Geometry check sheet. Reference: the model listing, model coordinates, mm. A direction names the side the tool comes from. Round coordinates to 2 decimals unless told otherwise and drop trailing zeros. Order: outer loops, then holes, each group sorted by start corner. A loop starts at its lowest first (then second) coordinate and runs counter-clockwise, first axis right, second up.
Autodesk Inventor part; units mm, degrees
ref_plane "YZ Plane" through (0, 0, 0) normal (1, 0, 0) x (0, 1, 0)
ref_plane "XZ Plane" through (0, 0, 0) normal (0, 1, 0) x (-1, 0, 0)
ref_plane "XY Plane" through (0, 0, 0) normal (0, 0, 1) x (1, 0, 0)
sketch "Sketch1" plane through (0, 0, 0) normal (0, 0, 1) x (1, 0, 0)
  line L0 (-107.95, -107.95) -> (107.95, -107.95)
  line L1 (107.95, -107.95) -> (107.95, 107.95)
  line L2 (107.95, 107.95) -> (-107.95, 107.95)
  line L3 (-107.95, 107.95) -> (-107.95, -107.95)
  line L4 (-107.95, -107.95) -> (107.95, 107.95) construction
  point P0 (0, 0)
  point P1 (0, 0)
  dimension "d0" = 215.9
  dimension "d1" = 215.9
extrude "Extrusion1" add sketch "Sketch1" along normal blind 6.35
sketch "Sketch3" plane through (0, 0, 6.35) normal (0, 0, 1) x (1, 0, 0)
  circle A0 centre (0, 0) radius 57.785
  dimension "d44" = 115.57
extrude "Extrusion3" cut sketch "Sketch3" against normal through all
sketch "Sketch5" plane through (0, 0, 6.35) normal (0, 0, 1) x (1, 0, 0)
  line L0 (-95.25, -95.25) -> (95.25, -95.25) construction
  line L1 (95.25, -95.25) -> (95.25, 95.25) construction
  line L2 (95.25, 95.25) -> (-95.25, 95.25) construction
  line L3 (-95.25, 95.25) -> (-95.25, -95.25) construction
  line L4 (-95.25, -95.25) -> (95.25, 95.25) construction
  point P0 (0, 0)
  point P1 (0, 0)
  point P2 (0, 0)
  dimension "d15" = 190.5
  dimension "d16" = 190.5
hole "Hole1" at (-95.25, 95.25, 6.35) at (95.25, 95.25, 6.35) at (95.25, -95.25, 6.35) at (-95.25, -95.25, 6.35) direction (0, 0, -1) diameter 4.4958 end through all counterbore diameter 7.9502 counterbore depth 4.1656
sketch "Sketch6" plane through (0, 0, 0) normal (0, 0, -1) x (-1, 0, 0)
  line L0 (-63.5, -63.5) -> (63.5, -63.5) construction
  line L1 (63.5, -63.5) -> (63.5, 63.5) construction
  line L2 (63.5, 63.5) -> (-63.5, 63.5) construction
  line L3 (-63.5, 63.5) -> (-63.5, -63.5) construction
  line L4 (-63.5, -63.5) -> (63.5, 63.5) construction
  point P0 (0, 0)
  point P1 (0, 0)
  dimension "d24" = 127
  dimension "d25" = 127
hole "Hole2" at (63.5, 63.5, 0) at (-63.5, 63.5, 0) at (-63.5, -63.5, 0) at (63.5, -63.5, 0) direction (0, 0, 1) diameter 3.302 end through all
sketch "Sketch7" plane through (0, 0, 6.35) normal (0, 0, 1) x (1, 0, 0)
  line L0 (-91.44, -91.44) -> (91.44, -91.44) construction
  line L1 (91.44, -91.44) -> (91.44, 91.44) construction
  line L2 (91.44, 91.44) -> (-91.44, 91.44) construction
  line L3 (-91.44, 91.44) -> (-91.44, -91.44) construction
  line L4 (-91.44, -91.44) -> (91.44, 91.44) construction
  line L5 (-151.13, 0) -> (151.13, 0) construction
  line L6 (0, -151.13) -> (0, 151.13) construction
  point P0 (0, 0)
  point P1 (0, 0)
  point P2 (-68.58, 91.44)
  point P3 (0, 91.44)
  point P4 (68.58, 91.44)
  point P5 (91.44, 68.58)
  point P6 (91.44, 0)
  point P7 (91.44, -68.58)
  point P8 (68.58, -91.44)
  point P9 (0, -91.44)
  point P10 (-68.58, -91.44)
  point P11 (-91.44, -68.58)
  point P12 (-91.44, 0)
  point P13 (-91.44, 68.58)
  dimension "d33" = 182.88
  dimension "d34" = 182.88
  dimension "d35" = 22.86
  dimension "d36" = 22.86
hole "Hole3" at (-68.58, 91.44, 6.35) at (0, 91.44, 6.35) at (68.58, 91.44, 6.35) at (91.44, 68.58, 6.35) at (91.44, 0, 6.35) at (91.44, -68.58, 6.35) at (68.58, -91.44, 6.35) at (0, -91.44, 6.35) at (-68.58, -91.44, 6.35) at (-91.44, -68.58, 6.35) at (-91.44, 0, 6.35) at (-91.44, 68.58, 6.35) direction (0, 0, -1) diameter 3.302 end through all
equation "\"d15\" = d16"
equation "\"d25\" = d24"
properties part number "J002448" material "ALUMINUM, 6061-T651"
(1) Draft check along Y on faces 3 (the flat face through (107.95, -2, 3)), 4 (the flat face through (-2, -107.95, 3)), 5 (the flat face through (-93.5, -97, 2.184)). Enter one of: released by +Y, released by -Y, zero draft, split by the parting line, or undercut.
Returned:
face 3: zero draft
face 4: released by -Y
face 5: undercut
(2) Set-up check for faces 1 (the cylindrical face through (-91.37, -94.39, 4.24)), 2 (the flat face through (-107.95, 2, 3)): record each of +Z, -Z, +X, -X, +Y, -Y from which the full face is reachable in a straight line by a thin tool's end or side.
Returned:
face 1: +Z
face 2: +Z, -Z, -X, +Y, -Y
(3) Sectioned sample at A-A, the plane x = 17. Record the cut outline in (y, z).
Returned:
outline: (-107.95, 0) - (-55.23, 0) - (-55.23, 6.35) - (-107.95, 6.35) - close; (55.23, 0) - (107.95, 0) - (107.95, 6.35) - (55.23, 6.35) - close
(4) Sectioned sample at B-B, the plane z = 4.5. Give the number of separate pieces and of enclosed holes in the cut face, and give its area (3 significant figures).
Returned:
separate pieces: 1
enclosed holes: 21
area: 35,800 mm2
(5) Depth check by flat-ended pin: P1, Ø6, axis at x = 95.25, y = -95.25, coming from the +Z side. Enter the tip coordinate at first touch or a pass-through.
Returned:
P1: stops at z = 2.18
(6) Material ranges on line 1 (X direction, y = 68.58, z = 3); line 2 (Y direction, x = 91.44, z = 1.5); line 3 (X direction, y = 95.25, z = 4.85), recorded low to high.
Returned:
line 1: x = -107.95 to -93.09, -89.79 to 89.79, 93.09 to 107.95
line 2: y = -107.95 to -70.23, -66.93 to -1.65, 1.65 to 66.93, 70.23 to 107.95
line 3: x = -107.95 to -99.23, -91.27 to 91.27, 99.23 to 107.95
